Autodesk Inventor part; units mm, degrees
ref_plane "YZ Plane" through (0, 0, 0) normal (1, 0, 0) x (0, 1, 0)
ref_plane "XZ Plane" through (0, 0, 0) normal (0, 1, 0) x (-1, 0, 0)
ref_plane "XY Plane" through (0, 0, 0) normal (0, 0, 1) x (1, 0, 0)
sketch "Náčrt1" plane through (0, 0, 0) normal (0, 0, 1) x (1, 0, 0)
  line L0 (0, 0) -> (16.9868, 0)
  line L1 (0, 17.5) -> (0, 35)
  line L2 (5, 23) -> (15, 23)
  line L3 (15, 23) -> (15, 12)
  line L4 (15, 12) -> (16.634, 12)
  line L5 (16.634, 12) -> (18.5, 11.5)
  line L6 (18.5, 11.5) -> (29, 11.5)
  line L7 (29, 11.5) -> (29, 8.5)
  line L8 (29, 8.5) -> (11, 8.5)
  line L9 (11, 8.5) -> (11, 17.5)
  line L10 (11, 17.5) -> (0, 17.5)
  line L11 (0, 35) -> (5, 35)
  line L12 (5, 35) -> (5, 23)
  dimension "d0" = 29
  dimension "d2" = 10.5
  dimension "d5" = 14
  dimension "d8" = 46
  dimension "d10" = 24
  dimension "d11" = 23
  dimension "d12" = 17
  dimension "d13" = 35
  dimension "d14" = 11
  dimension "d15" = 15
  dimension "d40" = 12.366
  dimension "d53" = 70
  dimension "d54" = 24
revolve "Rotace1" add sketch "Náčrt1" angle 360 about axis through (0, 0, 0) along (1, 0, 0)
chamfer "Zkosení3" distance 1 angle 45 1 edges at (15, -23, 0)
chamfer "Zkosení5" distance 1 angle 15 1 edges at (29, -11.5, 0) measured on face at (25.5, 11.4627, -0.9254)
chamfer "Zkosení6" distance 0.5 angle 45 1 edges at (0, -17.5, 0)
chamfer "Zkosení8" distance 1 angle 45 1 edges at (29, -8.5, 0)
chamfer "Zkosení9" distance 1 angle 45 1 edges at (11, -8.5, 0)
chamfer "Zkosení11" distance 1 angle 45 1 edges at (5, -35, 0)
chamfer "Zkosení12" distance 1 angle 45 1 edges at (0, -35, 0)
sketch "Náčrt3" plane through (0, 0, 0) normal (-1, 0, 0) x (0, 0, 1)
  line L0 (-39.3312, 12.9904) -> (-32.5, 12.9904)
  line L1 (-32.5, 12.9904) -> (-32.5, -12.9904)
  line L2 (-32.5, -12.9904) -> (-39.3312, -12.9904)
  line L3 (-39.3312, -12.9904) -> (-39.3312, 12.9904)
  line L4 (52.9331, 12.9904) -> (32.5, 12.9904)
  line L5 (32.5, 12.9904) -> (32.5, -12.9904)
  line L6 (32.5, -12.9904) -> (52.9331, -12.9904)
  line L7 (52.9331, -12.9904) -> (52.9331, 12.9904)
  line L8 (0, 0) -> (0, -6.1481) construction
  circle A0 centre (0, 0) radius 35 construction
  dimension "d61" = 65
extrude "Vysunutí2" cut sketch "Náčrt3" against normal through all
equation "\"Rozmer_B\" = 0"
equation "\"Rozmer_C\" = 0"
equation "\"Rozmer_D\" = d0"
properties part number "NA-45-h-Crown-247" material "12 060.4"
Read the model definition and answer for the solid it produces. Units are mm, in the model's axes. A direction names the side the tool comes from. Give positions to 0.01 mm unless a question says otherwise; leave off trailing zeros. Order: outer loops, then holes, each group sorted by start corner. A loop starts at its lowest first (then second) coordinate and runs counter-clockwise, first axis right, second up.
(1) For a pull along Y with two mould halves and no side action, classify faces 3 (the cylindrical face through (19.888, 4.57, -7.167)), 4 (the flat face through (11, 8, -8)), 5 (the flat face through (0, 15, -14)), 6 (the cylindrical face through (23.3, -1.5, 11.4)) as released by +Y, released by -Y, zero draft, split by the parting line, or undercut.
(2) For faces 1 (the conical face through (4.826, 34.168, 0.609)), 2 (the flat face through (15, 9, -9)), determine the directions among +Z, -Z, +X, -X, +Y, -Y from which every point of the face is accessible in a straight line to the end or side of a thin tool.
(3) Find section B-B (x = 21.5). Give the vertices of the cut face in (y, z), plus the area to 3 significant figures.
(4) Given pin 1 (2 mm diameter, centred on x = 13.5, z = 15.5, fed in from +Y); pin 2 (10 mm diameter, centred on y = 15.5, z = 19.5, fed in from +X); pin 3 (5 mm diameter, centred on x = 24, z = -0.5, fed in from -Y), each flat-ended and moving along its own axis, determine where each tip first touches the part or whether it passes through.
(5) Straight lines are drawn through the part: L1, parallel to Z at x = 4.75, y = 0; L2, parallel to Z at x = 22.5, y = 0; L3, parallel to X at y = 5.5, z = 19. For each, find the intervals that lie inside material, in ascending order.
Result sheet:
1. face 3: undercut
1. face 4: undercut
1. face 5: zero draft
1. face 6: split by the parting line
2. face 1: +X, +Y
2. face 2: +X
3. outline: circle Ø23 at (0, 0); hole circle Ø17 at (0, 0)
3. area: 188 mm2
4. pin 1: stops at y = 17.85
4. pin 2: stops at x = 15
4. pin 3: stops at y = -11.5
5. L1: z = -32.5 to -17.5, 17.5 to 32.5
5. L2: z = -11.5 to -8.5, 8.5 to 11.5
5. L3: x = 0 to 15
